Geometry: final body of the model. Coordinates: model frame, mm. Face numbers are marked on the shaded views. A direction names the side the tool comes from. Give positions to 0.01 mm unless a question says otherwise; leave off trailing zeros. Write each loop counter-clockwise with the first axis right and the second up, starting at its lowest first coordinate (ties: lowest second). Pieces come first, ordered by that corner, then holes.
Q1. Line query: line 1 (Y direction, x = -3.25, z = 5.75); line 2 (X direction, y = 4.25, z = 0); line 3 (X direction, y = 1.5, z = 0.75). Output: solid intervals per line, ascending.
Q2. Section A-A (x = 1.5). Return the cut outline in (y, z).
Q3. Section D-D (z = -7). Return the cut outline in (x, y).
Q4. Pin query (flat end, axial travel): pin 1 Ø1.5 at (x, y) = (-3.5, 3.5) entering from -Z; pin 2 Ø1.5 at (y, z) = (8.5, 5) entering from +X; pin 3 Ø1 at (y, z) = (7, -3) entering from -X. Return the tip coordinate at first contact, or that it passes through.
Q5. Reachability of the marked faces 5, 6 and 7 from +Z, -Z, +X, -X, +Y, -Y: full face, straight path, thin tool, end or side. Return the list, or none.
Q6. Mould query, pull axis Z, two halves, no side actions, for the marked faces 1, 2, 3 and 4. Classes: +Z half, -Z half, draft (parallel to the pull), parting line (faces both ways), or undercut.
Q7. Section B-B (y = 5.5). Return the cut outline in (x, z), plus the area to 3 significant figures.
Q8. Section C-C (z = 3). Return the cut outline in (x, y), plus the area to 3 significant figures.
from build123d import *

# Parameters (mm, degrees)
SKETCH_1_R          = 9
SKETCH_1_R_2        = 4
EXTRUDE_1_DEPTH     = 10
SKETCH_2_R          = 9.49914793
CUT_EXTRUDE_2_DEPTH = 6.5


with BuildPart() as part:
    # 草图1 → 拉伸1 (new body)
    with BuildSketch(Plane(origin=(0, 0, 0), x_dir=(1, 0, 0), z_dir=(0, 1, 0))):
        with Locations(Location((0, 0, 0), (0, 0, 270))):
            Circle(SKETCH_1_R)
        with Locations(Location((0, 0, 0), (0, 0, 270))):
            Circle(SKETCH_1_R_2, mode=Mode.SUBTRACT)
    extrude(amount=EXTRUDE_1_DEPTH)

    # 草图2 → 拉伸2 (cut)
    with BuildSketch(Plane(origin=(0, 10, 0), x_dir=(1, 0, 0), z_dir=(0, 1, 0))):
        Circle(SKETCH_2_R)
        Polygon((6.584703233, -3.602085044), (6.411848771, 3.901477754), (-0.172854462, 7.503562798), (-6.584703233, 3.602085044), (-6.411848771, -3.901477754), (0.172854462, -7.503562798), align=None, mode=Mode.SUBTRACT)
    extrude(amount=-CUT_EXTRUDE_2_DEPTH, mode=Mode.SUBTRACT)


solid = part.part
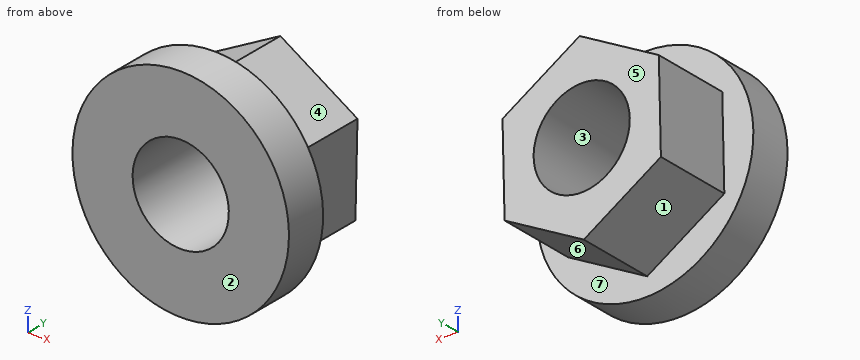
Computed:
1. line 1: y = 0 to 3.5
1. line 2: x = -6.5 to -4, 4 to 6.5
1. line 3: x = -8.97 to -3.93, 3.93 to 8.97
2. outline: (0, -8.87) - (3.5, -8.87) - (3.5, -6.59) - (10, -6.59) - (10, -3.71) - (0, -3.71) - close; (0, 3.71) - (10, 3.71) - (10, 6.7) - (3.5, 6.7) - (3.5, 8.87) - (0, 8.87) - close
3. outline: (-5.66, 0) - (5.66, 0) - (5.66, 3.5) - (0.75, 3.5) - (0.75, 10) - (-1, 10) - (-1, 3.5) - (-5.66, 3.5) - close
4. pin 1: stops at z = -8.57
4. pin 2: stops at x = 5.52
4. pin 3: stops at x = -6.58
5. face 5: +Z, -Z, +X, -X, +Y
5. face 6: -Z, +X, +Y
5. face 7: +Y
6. face 1: -Z half
6. face 2: draft
6. face 3: undercut
6. face 4: +Z half
7. outline: (-6.58, -3.6) - (-0.17, -7.5) - (6.41, -3.9) - (6.58, 3.6) - (0.17, 7.5) - (-6.41, 3.9) - close; hole circle Ø8 at (0, 0)
7. area: 96.1 mm2
8. outline: (-8.49, 0) - (-2.65, 0) - (-2.65, 10) - (-6.43, 10) - (-6.43, 3.5) - (-8.49, 3.5) - close; (2.65, 0) - (8.49, 0) - (8.49, 3.5) - (6.57, 3.5) - (6.57, 10) - (2.65, 10) - close
8. area: 91.0 mm2
